Input: part model. Units: mm. Frame: model coordinates. A direction names the side the tool comes from. Round coordinates to 2 decimals unless told otherwise and drop trailing zeros. Loops run counter-clockwise (first coordinate to the right, second up) from the corner with the lowest first, then second, coordinate; pieces in that order, holes last. Notation, with made-up numbers: (-39.5, -37) - (-9.5, -37) arc R28 cw to (-9.5, -5) - close; hole circle Ø11 at (52.25, -4). An arc over 180 degrees is marked (long way). One line per question, with ' | ' between items. Start each with the question number.
Item 1: Set-up query: faces 4 (the face through (-35, 2, 7.5)), 5 (the face through (1, 4.5, -3)). Return all of +Z, -Z, +X, -X, +Y, -Y with unobstructed straight access to the full face (end or side cutting, diameter ignored); none if empty.
Item 2: Draft query along Z for faces 1 (the face through (50, 2, -1)), 2 (the face through (35, 2, 14)), 3 (the face through (46, 2, -73.5)). Return one class per face: pulls with the +Z half, pulls with the -Z half, needs draft (parallel to the pull), parting line crosses it, or undercut.
Item 3: Section C-C, the plane x = -33. Return loops of the section in (y, z).
Item 4: Section D-D, the plane x = -13. Return loops of the section in (y, z), plus the area to 3 significant figures.
Item 5: Section B-B, the plane z = 15.5. Return loops of the section in (x, y), plus the area to 3 significant figures.
Item 6: First-contact query: pin 1 (1.3 mm diameter, centred on x = -46, y = 2, fed in from -Z); pin 2 (2 mm diameter, centred on y = 2.5, z = -75, fed in from +X). Flat tips, straight axial feed; report the tip coordinate or a pass-through.
Item 7: Section A-A, the plane z = -31.5. Return loops of the section in (x, y), plus the area to 3 significant figures.
Item 8: Material intervals for line 1 along Z through (x, y) = (38, 3.15); line 2 along Z through (x, y) = (-16, 2.4); line 3 along X through (y, z) = (3.2, -31.5), sorted ascending.
```python
from build123d import *

# Parameters (mm, degrees)
SKETCH2_W           = 40
SKETCH2_H           = 20
BOSS_EXTRUDE1_DEPTH = 4.5


with BuildPart() as part:
    # Sketch2 → Boss-Extrude1 (new body)
    with BuildSketch(Plane(origin=(0, 0, 0), x_dir=(1, 0, 0), z_dir=(0, 1, 0))):
        Polygon((-42, 73.5), (-42, 78), (42, 78), (42, 73.5), (50, 73.5), (50, -73.5), (-50, -73.5), (-50, 73.5), align=None)
        Polygon((-43, -4.5), (-43, -17), (-30, -17), (-30, -14), (-40, -14), (-40, -7.5), (-30, -7.5), (-30, -4.5), align=None, mode=Mode.SUBTRACT)
        Polygon((30, -17), (30, -14), (40, -14), (40, -7.5), (30, -7.5), (30, -4.5), (43, -4.5), (43, -17), align=None, mode=Mode.SUBTRACT)
        with Locations((0, 31.5)):
            Rectangle(SKETCH2_W, SKETCH2_H, mode=Mode.SUBTRACT)
    extrude(amount=BOSS_EXTRUDE1_DEPTH)


solid = part.part
```
Return value:
1) face 4: +Y, -Y | face 5: +Z, -Z, +X, -X, +Y
2) face 1: needs draft | face 2: undercut | face 3: pulls with the -Z half
3) outline: (0, -78) - (4.5, -78) - (4.5, 4.5) - (0, 4.5) - close; (0, 7.5) - (4.5, 7.5) - (4.5, 14) - (0, 14) - close; (0, 17) - (4.5, 17) - (4.5, 73.5) - (0, 73.5) - close
4) outline: (0, -78) - (4.5, -78) - (4.5, -41.5) - (0, -41.5) - close; (0, -21.5) - (4.5, -21.5) - (4.5, 73.5) - (0, 73.5) - close | area: 592 mm2
5) outline: (-50, 0) - (-43, 0) - (-43, 4.5) - (-50, 4.5) - close; (-30, 0) - (30, 0) - (30, 4.5) - (-30, 4.5) - close; (43, 0) - (50, 0) - (50, 4.5) - (43, 4.5) - close | area: 333 mm2
6) pin 1: z = -73.5 | pin 2: x = 42
7) outline: (-50, 0) - (-20, 0) - (-20, 4.5) - (-50, 4.5) - close; (20, 0) - (50, 0) - (50, 4.5) - (20, 4.5) - close | area: 270 mm2
8) line 1: -78 to 4.5, 7.5 to 14, 17 to 73.5 | line 2: -78 to -41.5, -21.5 to 73.5 | line 3: -50 to -20, 20 to 50
